Model file for the job. Use its own axes, mm. Coordinates: 2 decimals unless noted, no trailing zeros. Order: outer loops, then holes, each group sorted by start corner. A loop starts at its lowest first (then second) coordinate and runs counter-clockwise, first axis right, second up. Notation, with made-up numbers: (-5, 29) -> (10, 29) arc R22 ccw to (10, 48) -> close; hole circle Ø2 at (28.25, 7.25). An arc over 180 degrees is marked (long way). Return JSON: item names as keys, results as strings. Group by question number.
1) Cut at A-A (x = -34). Write the cut outline in (y, z).
2) Cut at C-C (z = 5.25). Write the cut outline in (x, y).
3) Pull direction Y, two halves, no side cores. Call faces 1 (the cylindrical face through (-30.424, -13.149, 4.056)), 2 (the flat face through (99, -190, 4)), 3 (the flat face through (95.5, -88.81, 3.94)), 4 (the cylindrical face through (93.474, -158.484, 4.056)): +Y half, -Y half, draft (parallel to the pull), parting line (faces both ways), or undercut.
4) Cut at B-B (y = -12). Write the cut outline in (x, z), and give its area (3 significant figures).
5) Flat gauge pins, fed straight in: pin 1 (1 mm diameter, centred on y = -102.5, z = 2.5, fed in from +X); pin 2 (8 mm diameter, centred on x = 68.23, y = -155.07, fed in from +Z); pin 3 (2 mm diameter, centred on x = 125.5, z = 2.5, fed in from +Y); pin 4 (1 mm diameter, centred on x = -23, z = 5, fed in from -Y). Where does each tip first touch, or does it go through?
6) Probe line 1 (X direction, y = -179, z = 2.75); line 2 (X direction, y = -9.5, z = 6); line 3 (Y direction, x = 70, z = 2.5). List the from-to ranges inside material, lowest first.
7) Cut at D-D (y = -179). Write the cut outline in (x, z), and give its area (3 significant figures).
from build123d import *

# Parameters (mm, degrees)
BOSS_EXTRU_1_DEPTH      = 8
ESQUISSE2_R             = 3
ESQUISSE2_R_2           = 3.5
ENL_V_MAT_EXTRU_1_DEPTH = 644.25917494


with BuildPart() as part:
    # Esquisse1 → Boss.-Extru.1 (new body)
    with BuildSketch(Plane.XY):
        with BuildLine():
            Line((-38.452994616, 0), (38.452994616, 0))
            ThreePointArc((38.452994616, 0), (43.452994616, -1.339745962), (47.113248654, -5))
            Line((47.113248654, -5), (145.262794416, -175))
            ThreePointArc((145.262794416, -175), (145.262794416, -185), (136.602540378, -190))
            Line((136.602540378, -190), (59.696551146, -190))
            ThreePointArc((59.696551146, -190), (54.696551146, -188.660254038), (51.036297108, -185))
            Line((51.036297108, -185), (-47.113248654, -15))
            ThreePointArc((-47.113248654, -15), (-47.113248654, -5), (-38.452994616, 0))
        make_face()
    extrude(amount=BOSS_EXTRU_1_DEPTH)

    # Esquisse2 → Enlèv. mat.-Extru.1 (cut, through all)
    with BuildSketch(Plane(origin=(81.232648941, -630, 8), x_dir=(1, 0, 0), z_dir=(0, 0, 1))):
        with Locations((-114.42794679, 618)):
            Circle(ESQUISSE2_R)
        with Locations((-64.42794679, 618)):
            Circle(ESQUISSE2_R)
        with Locations((-13, 474.932525236)):
            Circle(ESQUISSE2_R_2)
        with Locations((13, 474.932525236)):
            Circle(ESQUISSE2_R_2)
        with Locations((-18.010451836, 451)):
            Circle(ESQUISSE2_R)
        with Locations((50.751089284, 451)):
            Circle(ESQUISSE2_R)
    extrude(amount=-ENL_V_MAT_EXTRU_1_DEPTH, mode=Mode.SUBTRACT)


solid = part.part
Answers below:
{
 "1": {"outline": "(-37.71, 0) -> (-14.89, 0) -> (-14.89, 8) -> (-37.71, 8) -> close; (-9.11, 0) -> (0, 0) -> (0, 8) -> (-9.11, 8) -> close"},
 "2": {"outline": "(-47.11, -15) -> (51.04, -185) arc R10 ccw to (59.7, -190) -> (136.6, -190) arc R10 ccw to (145.26, -175) -> (47.11, -5) arc R10 ccw to (38.45, 0) -> (-38.45, 0) arc R10 ccw to start; hole circle Ø6 at (-33.2, -12); hole circle Ø6 at (16.8, -12); hole circle Ø6 at (63.22, -179); hole circle Ø7 at (68.23, -155.07); hole circle Ø7 at (94.23, -155.07); hole circle Ø6 at (131.98, -179)"},
 "3": {"face 1": "undercut", "face 2": "-Y half", "face 3": "+Y half", "face 4": "undercut"},
 "4": {"outline": "(-48.25, 0) -> (-36.2, 0) -> (-36.2, 8) -> (-48.25, 8) -> close; (-30.2, 0) -> (13.8, 0) -> (13.8, 8) -> (-30.2, 8) -> close; (19.8, 0) -> (51.15, 0) -> (51.15, 8) -> (19.8, 8) -> close", "area": "699 mm^2"},
 "5": {"pin 1": "stops at x = 103.69", "pin 2": "stops at z = 8", "pin 3": "stops at y = -139.04", "pin 4": "stops at y = -57.63"},
 "6": {"line 1": "x = 47.57 to 60.22, 66.22 to 128.98, 134.98 to 146.55", "line 2": "x = -48.44 to -34.85, -31.54 to 15.15, 18.46 to 49.71", "line 3": "y = -190 to -158.09, -152.05 to -44.64"},
 "7": {"outline": "(47.57, 0) -> (60.22, 0) -> (60.22, 8) -> (47.57, 8) -> close; (66.22, 0) -> (128.98, 0) -> (128.98, 8) -> (66.22, 8) -> close; (134.98, 0) -> (146.55, 0) -> (146.55, 8) -> (134.98, 8) -> close", "area": "696 mm^2"}
}
